For this review, take the finished solid that the model builds, in its own axes (mm). Face numbers are marked on the shaded views. A direction names the side the tool comes from. Give positions to 0.01 mm unless a question says otherwise; leave off trailing zeros. Order: outer loops, then holes, each group sorted by start corner. A loop starts at its lowest first (then second) coordinate and runs counter-clockwise, first axis right, second up. Notation, with made-up numbers: (77.25, -10.5) -> (131.25, -10.5) arc R24 cw to (131.25, 10.5) -> close; hole circle Ø9 at (-30, 1.5). An arc over 180 degrees is marked (long way). Return JSON: item names as keys, results as strings. Group by question number.
1) Add section B-B (y = 8.5). Give the boundary of the cut face in (x, z).
2) Add section A-A (x = -2). Give the boundary of the cut face in (y, z).
3) For the marked faces 4 and 5, list the 3-axis set-ups (+Z, -Z, +X, -X, +Y, -Y) from which the entire face can be reached by the end or side of a thin tool; tool diameter is ignored.
4) To check wall thickness, follow line 1 along X through (y, z) = (-2, 63); line 2 along Y through (x, z) = (-22, 35); line 3 along Y through (x, z) = (4.5, 66). State the ranges of each line that lie inside material, in increasing order.
5) Insertion check: P1, Ø10, axis at x = -23.5, z = 54.5, coming from the -Y side; P2, Ø12, axis at y = -9.5, z = 25.5, coming from the +X side; P3, Ø8, axis at y = 8, z = 45, coming from the -X side. Each pin has a flat end and moves straight along its axis. Give the tip position at first contact, or say it passes through.
6) The part is to be moulded in two halves that separate along Y. For the marked faces 1, 2 and 3, say which applies: released by +Y, released by -Y, zero draft, split by the parting line, or undercut.
from build123d import *

# Parameters (mm, degrees)
F0_R     = 6.35
F1_DEPTH = 76.2


with BuildPart() as f1:
    # F0 (on Top) → F1 (new body)
    with BuildSketch(Plane.XY):
        with BuildLine():
            Line((-43.806983, -25.361842), (-44.06456, -25.27755))
            ThreePointArc((-44.06456, -25.27755), (-36.318587, -35.519013), (-26.252069, -43.49102))
            Line((-26.252069, -43.49102), (-21.279346, -46.128401))
            Line((-21.279346, -46.128401), (-4.724133, -54.908783))
            Line((-4.724133, -54.908783), (-22.398102, -35.196542))
            Line((-22.398102, -35.196542), (-17.613461, -30.90664))
            Line((-17.613461, -30.90664), (0.060508, -50.618881))
            Line((0.060508, -50.618881), (-0.14128, -50.799804))
            ThreePointArc((-0.14128, -50.799804), (12.057786, -49.34825), (23.551673, -45.010651))
            Line((23.551673, -45.010651), (29.977489, -41.012073))
            Line((29.977489, -41.012073), (45.190335, -31.545611))
            Line((45.190335, -31.545611), (19.28448, -36.995084))
            Line((19.28448, -36.995084), (17.959204, -30.707025))
            Line((17.959204, -30.707025), (43.867491, -25.257039))
            Line((43.867491, -25.257039), (43.92328, -25.522254))
            ThreePointArc((43.92328, -25.522254), (49.294753, -12.274661), (50.762755, 1.944916))
            Line((50.762755, 1.944916), (51.130101, 0))
            Line((51.130101, 0), (50.202441, 23.225819))
            Line((50.202441, 23.225819), (41.644922, -1.83064))
            Line((41.644922, -1.83064), (35.537437, 0.168029))
            Line((35.537437, 0.168029), (43.771755, 25.330256))
            Line((43.771755, 25.330256), (44.094956, 25.224489))
            ThreePointArc((44.094956, 25.224489), (35.237916, 36.591383), (23.545425, 45.01392))
            Line((23.545425, 45.01392), (4.688904, 54.877198))
            Line((4.688904, 54.877198), (22.362902, 35.164925))
            Line((22.362902, 35.164925), (17.578261, 30.875022))
            Line((17.578261, 30.875022), (-0.095736, 50.587295))
            Line((-0.095736, 50.587295), (0.14128, 50.799804))
            ThreePointArc((0.14128, 50.799804), (-14.048748, 48.818774), (-27.121244, 42.954373))
            Line((-27.121244, 42.954373), (-45.190335, 31.545611))
            Line((-45.190335, 31.545611), (-19.284156, 37.005613))
            Line((-19.284156, 37.005613), (-17.959204, 30.707025))
            Line((-17.959204, 30.707025), (-43.867491, 25.257039))
            Line((-43.867491, 25.257039), (-43.92328, 25.522254))
            ThreePointArc((-43.92328, 25.522254), (-49.304707, 12.234617), (-50.759528, -2.02738))
            Line((-50.759528, -2.02738), (-50.373884, -11.682765))
            Line((-50.373884, -11.682765), (-49.907264, -23.36553))
            Line((-49.907264, -23.36553), (-41.68015, 1.799054))
            Line((-41.68015, 1.799054), (-35.572666, -0.199615))
            Line((-35.572666, -0.199615), (-43.806983, -25.361842))
        make_face()
        Circle(F0_R, mode=Mode.SUBTRACT)
    extrude(amount=F1_DEPTH)


solid = f1.part
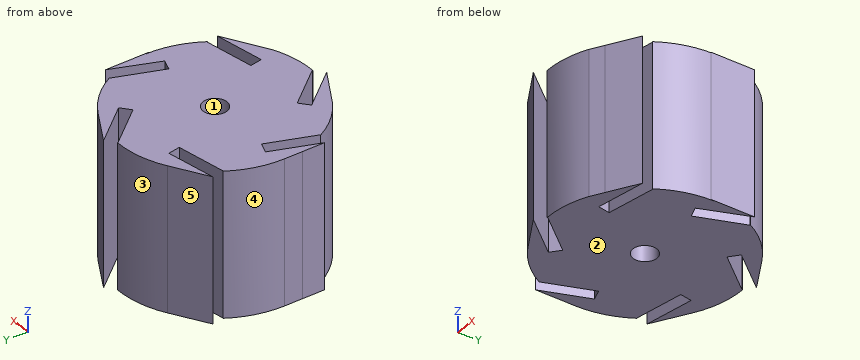
Evaluation:
{
 "1": {"outline": "(-50.08, 0) -> (38.26, 0) -> (38.26, 76.2) -> (-50.08, 76.2) -> close; (45.17, 0) -> (50.79, 0) -> (50.79, 76.2) -> (45.17, 76.2) -> close"},
 "2": {"outline": "(-48.32, 0) -> (-6.03, 0) -> (-6.03, 76.2) -> (-48.32, 76.2) -> close; (6.03, 0) -> (50.76, 0) -> (50.76, 76.2) -> (6.03, 76.2) -> close"},
 "3": {"face 4": "+Z, -Z, -X", "face 5": "+Z, -Z, -X, +Y"},
 "4": {"line 1": "-50.76 to -42.92, -36.16 to -6.03, 6.03 to 50.76", "line 2": "-45.75 to -35.64, -34.84 to 29.86, 36.43 to 45.79", "line 3": "-50.6 to -4.48, 4.48 to 45.46"},
 "5": {"P1": "y = -47.6", "P2": "x = 50.68", "P3": "x = -50.64"},
 "6": {"face 1": "undercut", "face 2": "zero draft", "face 3": "released by +Y"}
}
